Read the model definition and answer for the solid it produces. Units are mm, in the model's axes. Face numbers are marked on the shaded views. A direction names the side the tool comes from. Round coordinates to 2 decimals unless told otherwise and drop trailing zeros. Write each loop counter-clockwise with the first axis right and the second up, starting at its lowest first coordinate (ties: lowest second). Pieces come first, ordered by that corner, then holes. Notation, with made-up numbers: M 7,64 L 57,64 A16 cw 57,69 Z; hole C -4,28.25 d4. An arc over 180 degrees is marked long. Use one line per item in the form item = value. Start each with the question number.
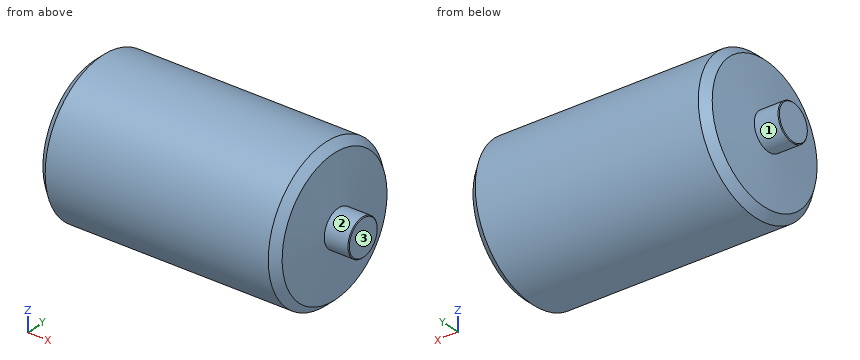
```python
from build123d import *

# Parameters (mm, degrees)
F2_SIZE  = 5
F3_SIZE  = 5
F4_SIZE2 = 0.5
F4_SIZE  = 0.5


with BuildPart() as f1:
    # F0 (on Top) → F1 (revolve)
    with BuildSketch(Plane.XY):
        Polygon((0, 12.5), (0, 0), (200, 0), (200, 12.5), (183.5, 12.5), (180.219175, 50), (19.780825, 50), (16.5, 12.5), align=None)
    revolve(axis=Axis((100, 0, 0), (1, 0, 0)))

    # F2
    f2_edges = [f1.edges().sort_by_distance(p)[0] for p in [
        (19.780825, -50, 0),
    ]]
    chamfer(f2_edges, length=F2_SIZE)

    # F3
    f3_edges = [f1.edges().sort_by_distance(p)[0] for p in [
        (180.219175, -50, 0),
    ]]
    chamfer(f3_edges, length=F3_SIZE)

    # F4
    f4_edges = [f1.edges().sort_by_distance(p)[0] for p in [
        (0, -12.5, 0),
        (200, -12.5, 0),
    ]]
    chamfer(f4_edges, length=F4_SIZE, length2=F4_SIZE2)


solid = f1.part
```
Q1. Find section A-A on x = 52. Write down the section's boundary in (y, z).
Q2. Straight lines are drawn through the part: line 1 (Y direction, x = 142, z = -30); line 2 (Y direction, x = 140, z = 22); line 3 (X direction, y = -14.5, z = 33.5). For each, find the intervals that lie inside material, in ascending order. Write a range as [from, to].
Q3. A tool of negligible diameter and unlimited length cuts with its end or side. For the marked faces 1, 2 and 3, from which of +Z, -Z, +X, -X, +Y, -Y can it reach the whole face along a straight path? Write none if from no direction.
Q4. Each of these flat-tipped pins is pushed along its axis until it touches: pin 1 Ø12 at (y, z) = (-26.5, -6) entering from -X; pin 2 Ø8 at (x, z) = (77, -9) entering from +Y; pin 3 Ø10 at (x, y) = (73.5, 26) entering from -Z; pin 4 Ø12 at (y, z) = (1.5, 17) entering from +X. Where does it stop, or does it pass through?
Response:
q1.outline = C 0,0 d100
q2.line_1 = [-40, 40]
q2.line_2 = [-44.9, 44.9]
q2.line_3 = [18.6, 181.4]
q3.face_1 = -X
q3.face_2 = +X
q3.face_3 = +Z, -Z, +X, +Y, -Y
q4.pin_1 = 17.26
q4.pin_2 = 49.75
q4.pin_3 = -45.38
q4.pin_4 = 200
